from build123d import *

# Parameters (mm, degrees)
F0_R        = 1.6
F0_R_2      = 3
F1_DEPTH    = 4
F2_T1_DEPTH = 4
F3_R        = 2.4


# Not quite as in the source:
# - a fillet or chamfer that OpenCascade refuses, or shapes differently, is made with other operations: its cross-section is extruded or revolved along the edge and cut away or added


with BuildPart() as f1:
    # F0 (on Top) → F1 (new body)
    with BuildSketch(Plane.XY):
        with BuildLine():
            ThreePointArc((80.3055021759, 68.9917936769), (73.1855518528, 73.1855518528), (68.9917936769, 80.3055021759))
            Line((68.9917936769, 80.3055021759), (1, 12.313708499))
            Line((1, 12.313708499), (0, 11.313708499))
            Line((0, 11.313708499), (0, 0))
            Line((0, 0), (11.313708499, 0))
            Line((11.313708499, 0), (12.313708499, 1))
            Line((12.313708499, 1), (80.3055021759, 68.9917936769))
        make_face()
        with Locations((4, 4)):
            Circle(F0_R, mode=Mode.SUBTRACT)
        with Locations((15.25, 15.25)):
            Circle(F0_R_2, mode=Mode.SUBTRACT)
        with Locations((26.499998178, 26.499998178)):
            Circle(F0_R, mode=Mode.SUBTRACT)
        with BuildLine():
            ThreePointArc((87.7873068843, 81.9183206005), (81.9183206005, 81.9183206005), (81.9183206005, 87.7873068843))
            Line((81.9183206005, 87.7873068843), (79.1959594929, 90.5096679919))
            Line((79.1959594929, 90.5096679919), (75.1224322345, 86.4361407335))
            ThreePointArc((75.1224322345, 86.4361407335), (75.2373217206, 86.4486400465), (75.3528137424, 86.4528137424))
            Line((75.3528137424, 86.4528137424), (76.8528137424, 86.4528137424))
            ThreePointArc((76.8528137424, 86.4528137424), (77.9841845923, 85.9841845923), (78.4528137424, 84.8528137424))
            ThreePointArc((78.4528137424, 84.8528137424), (77.9841845923, 83.7214428925), (76.8528137424, 83.2528137424))
            Line((76.8528137424, 83.2528137424), (75.3528137424, 83.2528137424))
            ThreePointArc((75.3528137424, 83.2528137424), (74.1427289494, 83.8060593329), (73.7694867513, 85.0831952502))
            Line((73.7694867513, 85.0831952502), (68.9917936769, 80.3055021759))
            ThreePointArc((68.9917936769, 80.3055021759), (73.1855518528, 73.1855518528), (80.3055021759, 68.9917936769))
            Line((80.3055021759, 68.9917936769), (85.0831952502, 73.7694867513))
            ThreePointArc((85.0831952502, 73.7694867513), (83.8060593329, 74.1427289494), (83.2528137424, 75.3528137424))
            Line((83.2528137424, 75.3528137424), (83.2528137424, 76.8528137424))
            ThreePointArc((83.2528137424, 76.8528137424), (84.8528137424, 78.4528137424), (86.4528137424, 76.8528137424))
            Line((86.4528137424, 76.8528137424), (86.4528137424, 75.3528137424))
            ThreePointArc((86.4528137424, 75.3528137424), (86.4486400465, 75.2373217206), (86.4361407335, 75.1224322345))
            Line((86.4361407335, 75.1224322345), (90.5096679919, 79.1959594929))
            Line((90.5096679919, 79.1959594929), (87.7873068843, 81.9183206005))
        make_face()
        with BuildLine():
            Line((79.1959594929, 90.5096679919), (81.9183206005, 87.7873068843))
            ThreePointArc((81.9183206005, 87.7873068843), (86.4409499867, 88.6869138023), (89.0028137424, 84.8528137424))
            ThreePointArc((89.0028137424, 84.8528137424), (88.6869138023, 83.2646774981), (87.7873068843, 81.9183206005))
            Line((87.7873068843, 81.9183206005), (90.5096679919, 79.1959594929))
            Line((90.5096679919, 79.1959594929), (86.4361407335, 75.1224322345))
            ThreePointArc((86.4361407335, 75.1224322345), (85.9841845923, 74.2214428925), (85.0831952502, 73.7694867513))
            Line((85.0831952502, 73.7694867513), (80.3055021759, 68.9917936769))
            ThreePointArc((80.3055021759, 68.9917936769), (83.083856654, 68.4479123157), (85.9142893623, 68.3869924902))
            add(Edge.make_bspline(
                [(101.3186349946, 83.7913381225), (90.8947856118, 78.810841873), (85.9142893623, 68.3869924902)],
                knots=[3.9431649716, 3.9431649716, 3.9431649716, 5.4816129892, 5.4816129892, 5.4816129892], degree=2, weights=[1, 0.7184506482, 1]))
            ThreePointArc((101.3186349946, 83.7913381225), (101.3442668418, 84.321800871), (101.3528137424, 84.8528137424))
            ThreePointArc((101.3528137424, 84.8528137424), (96.1385492583, 96.8895148629), (83.7913381225, 101.3186349946))
            add(Edge.make_bspline(
                [(68.3869924902, 85.9142893623), (78.810841873, 90.8947856118), (83.7913381225, 101.3186349946)],
                knots=[0.801572318, 0.801572318, 0.801572318, 2.3400203356, 2.3400203356, 2.3400203356], degree=2, weights=[1, 0.7184506482, 1]))
            ThreePointArc((68.3869924902, 85.9142893623), (68.4479123157, 83.083856654), (68.9917936769, 80.3055021759))
            Line((68.9917936769, 80.3055021759), (73.7694867513, 85.0831952502))
            ThreePointArc((73.7694867513, 85.0831952502), (74.2214428925, 85.9841845923), (75.1224322345, 86.4361407335))
            Line((75.1224322345, 86.4361407335), (79.1959594929, 90.5096679919))
        make_face()
        with BuildLine():
            ThreePointArc((95.9528137424, 84.8528137424), (95.4841845923, 83.7214428925), (94.3528137424, 83.2528137424))
            Line((94.3528137424, 83.2528137424), (92.8528137424, 83.2528137424))
            ThreePointArc((92.8528137424, 83.2528137424), (91.2528137424, 84.8528137424), (92.8528137424, 86.4528137424))
            Line((92.8528137424, 86.4528137424), (94.3528137424, 86.4528137424))
            ThreePointArc((94.3528137424, 86.4528137424), (95.4841845923, 85.9841845923), (95.9528137424, 84.8528137424))
        make_face(mode=Mode.SUBTRACT)
        with BuildLine():
            Line((83.2528137424, 92.8528137424), (83.2528137424, 94.3528137424))
            ThreePointArc((83.2528137424, 94.3528137424), (84.8528137424, 95.9528137424), (86.4528137424, 94.3528137424))
            Line((86.4528137424, 94.3528137424), (86.4528137424, 92.8528137424))
            ThreePointArc((86.4528137424, 92.8528137424), (84.8528137424, 91.2528137424), (83.2528137424, 92.8528137424))
        make_face(mode=Mode.SUBTRACT)
        Polygon((12.313708499, 0), (12.313708499, 1), (11.313708499, 0), align=None)
        Polygon((0, 11.313708499), (1, 12.313708499), (0, 12.313708499), align=None)
    extrude(amount=F1_DEPTH)

    # F2: fillet of radius 17.7 on 2 edges, made by hand

    # F2_s2 → F2_t1 (join)
    with BuildSketch(Plane.XY):
        with BuildLine():
            ThreePointArc((74.55426567, 63.240557171), (79.7659943294, 66.8474433344), (85.9142893623, 68.3869924902))
            ThreePointArc((85.9142893623, 68.3869924902), (83.083856654, 68.4479123157), (80.3055021759, 68.9917936769))
            Line((80.3055021759, 68.9917936769), (74.55426567, 63.240557171))
        make_face()
        with BuildLine():
            ThreePointArc((68.3869924902, 85.9142893623), (66.8474433344, 79.7659943294), (63.240557171, 74.55426567))
            Line((63.240557171, 74.55426567), (68.9917936769, 80.3055021759))
            ThreePointArc((68.9917936769, 80.3055021759), (68.4479123157, 83.083856654), (68.3869924902, 85.9142893623))
        make_face()
    extrude(amount=F2_T1_DEPTH)

    # F3
    f3_edges = [f1.edges().sort_by_distance(p)[0] for p in [
        (12.313708, 1, 2),
        (1, 12.313708, 2),
    ]]
    fillet(f3_edges, radius=F3_R)


solid = f1.part
Could you check a few things on this model? Use its own coordinates, in mm. A direction names the side the tool comes from. Give positions to 0.01 mm unless a question says otherwise; leave off trailing zeros. Order: outer loops, then holes, each group sorted by start corner. A loop starts at its lowest first (then second) coordinate and runs counter-clockwise, first axis right, second up.
Item 1: For faces 1 (the face through (84.888, 91.253, 1.972)), 2 (the face through (66.884, 79.847, 1.972)), which set-ups out of +Z, -Z, +X, -X, +Y, -Y let a thin tool reach every point of the face, with its end or its side?
Item 2: If we mould it in two halves opening along X, with no side actions, what happens to faces 3 (the face through (32.903, 44.216, 1.972)), 4 (the face through (50, 55, 0)), 5 (the face through (84.818, 78.452, 1.972))? For each: pulls with the +X half, pulls with the -X half, needs draft (parallel to the pull), parting line crosses it, or undercut.
Item 3: If we section it at D-D, the plane y = 66.5: Write out the boundary of the cut face in (x, z).
Item 4: If we section it at C-C, the plane z = 1.3: Count the separate pieces of the cut face and the enclosed holes in it, plus the area to 3 significant figures.
Item 5: I need wall thicknesses on line 1 (Y direction, x = 78, z = 2.4); line 2 (Y direction, x = 4, z = 1.05); line 3 (X direction, y = 83, z = 1.5). Which ranges of each line are inside material? Lowest first, please.
Item 6: If we section it at A-A, the plane y = 15.25: Write out the boundary of the cut face in (x, z).
Item 7: I'm going to push flat-ended pins straight in: pin 1 (1.5 mm diameter, centred on y = 36.5, z = 2.5, fed in from -X); pin 2 (0.8 mm diameter, centred on x = 76, z = 2.5, fed in from -Y); pin 3 (1.2 mm diameter, centred on y = 76.5, z = 2, fed in from -X) (3 decimals); pin 4 (2.5 mm diameter, centred on x = 26.5, y = 26.5, fed in from -Z). Where does each tip first touch, or does it pass through?
Values:
1. face 1: +Z, -Z
1. face 2: +Z, -Z, -X, +Y
2. face 3: pulls with the -X half
2. face 4: needs draft
2. face 5: undercut
3. outline: (55.19, 0) - (79.04, 0) - (79.04, 4) - (55.19, 4) - close
4. separate pieces: 1
4. enclosed holes: 8
4. area: 2,150 mm2
5. line 1: y = 65.92 to 83.74, 85.97 to 93.27
5. line 2: y = 0 to 2.4, 5.6 to 15.31
5. line 3: x = 67.95 to 81.14, 88.57 to 99.82
6. outline: (3.94, 0) - (12.25, 0) - (12.25, 4) - (3.94, 4) - close; (18.25, 0) - (26.56, 0) - (26.56, 4) - (18.25, 4) - close
7. pin 1: stops at x = 24.44
7. pin 2: stops at y = 64.21
7. pin 3: stops at x = 64.455
7. pin 4: passes through
